Input: part model. Units: mm. Frame: model coordinates. A direction names the side the tool comes from. Give positions to 0.01 mm unless a question says otherwise; leave off trailing zeros. Write each loop counter-clockwise with the first axis right and the second up, starting at its lowest first coordinate (ties: lowest second). Pieces come first, ordered by that corner, then holes. Notation, with made-up numbers: (89, 14.5) - (121, 14.5) arc R22 cw to (121, 23.5) - close; hole circle Ø11 at (85.25, 72.5). An arc over 180 degrees is marked (long way). Answer as CSV lines item,"result".
```python
from build123d import *

# Parameters (mm, degrees)
BOSS_EXTRUDE4_DEPTH      = 4.2
BOSS_EXTRUDE4_DEPTH_BACK = 0.2
SKETCH10_R               = 5
BOSS_EXTRUDE5_DEPTH      = 9
SKETCH16_R               = 5
BOSS_EXTRUDE6_DEPTH      = 4.8
CUT_EXTRUDE2_DEPTH       = 20.805049861
HOLEWZD2_D               = 3.5
HOLEWZD2_DEPTH           = 1.8
CHAMFER2_SIZE            = 0.4


with BuildPart() as part:
    # Sketch10 → Boss-Extrude4 (new, two sides: drawn at the far end of the back side and taken through both)
    with BuildSketch(Plane.XY.offset(0.4).offset(-BOSS_EXTRUDE4_DEPTH_BACK)):
        with Locations((1, 0)):
            Circle(SKETCH10_R)
    extrude(amount=BOSS_EXTRUDE4_DEPTH + BOSS_EXTRUDE4_DEPTH_BACK)

    # Sketch11 → Boss-Extrude5 (add)
    with BuildSketch(Plane(origin=(0, 0, 0.2), x_dir=(-1, 0, 0), z_dir=(0, 0, -1))):
        with BuildLine():
            Line((-4, -3.05), (-4, 3.05))
            ThreePointArc((-4, 3.05), (-3.824264069, 3.474264069), (-3.4, 3.65))
            Line((-3.4, 3.65), (0, 3.65))
            ThreePointArc((0, 3.65), (3.65, 0), (0, -3.65))
            Line((0, -3.65), (-3.4, -3.65))
            ThreePointArc((-3.4, -3.65), (-3.824264069, -3.474264069), (-4, -3.05))
        make_face()
    extrude(amount=BOSS_EXTRUDE5_DEPTH)

    # Sketch16 → Boss-Extrude6 (add)
    with BuildSketch(Plane(origin=(0, 0, 4.6), x_dir=(-1, 0, 0), z_dir=(0, 0, -1))):
        with Locations((1, 0)):
            Circle(SKETCH16_R)
    extrude(amount=-BOSS_EXTRUDE6_DEPTH)

    # Sketch17 → Cut-Extrude2 (cut, through all)
    with BuildSketch(Plane.XY.offset(9.4)):
        with BuildLine():
            Line((2.2, -1.47732867), (2.2, 1.47732867))
            ThreePointArc((2.2, 1.47732867), (-2.65, 0), (2.2, -1.47732867))
        make_face()
    extrude(amount=-CUT_EXTRUDE2_DEPTH, mode=Mode.SUBTRACT)

    # HoleWzd2
    with Locations(Plane(origin=(4, 0, 0), x_dir=(0, 0, -1), z_dir=(1, 0, 0))):
        with Locations((5, 0)):
            Hole(HOLEWZD2_D / 2, depth=HOLEWZD2_DEPTH)

    # Chamfer2
    # the kernel refuses this chamfer: 0.4 mm, written as the material it takes off along each edge
    with BuildSketch(Plane(origin=(-1, 0, 9.4), x_dir=(-1, 0, 0), z_dir=(0, -1, 0))) as chamfer2_piece_1:
        Polygon((5, CHAMFER2_SIZE), (5 - CHAMFER2_SIZE, 0), (5, 0), align=None)
    revolve(axis=Axis((-1, 0, 9.4), (0, 0, -1)), mode=Mode.SUBTRACT)
    with BuildSketch(Plane(origin=(1, 0, 0.2), x_dir=(1, 0, 0), z_dir=(0, -1, 0))) as chamfer2_piece_2_section:
        Polygon((5, CHAMFER2_SIZE), (5 - CHAMFER2_SIZE, 0), (5, 0), align=None)
    chamfer2_piece_2 = revolve(axis=Axis((1, 0, 0.2), (0, 0, 1)), mode=Mode.PRIVATE)
    chamfer2_piece_2 = chamfer2_piece_2 - Plane(origin=(0, 0, 0.390166904), x_dir=(0, 1, 0), z_dir=(0, 0, 1)) * Cylinder(3.65, 20, mode=Mode.PRIVATE)
    add(chamfer2_piece_2, mode=Mode.SUBTRACT)


solid = part.part
```
Item 1: Mould query, pull axis Y, two halves, no side actions, for faces 1 (the face through (5.77, 1.5, 2.57)), 2 (the face through (3, 0, -8.8)), 3 (the face through (2.2, 0, 3)). Classes: +Y half, -Y half, draft (parallel to the pull), parting line (faces both ways), or undercut.
The answers:
face 1,"parting line"
face 2,"draft"
face 3,"undercut"
Item 2: Contact query for flat-ended pins moving along their axis: pin 1 (5.5 mm diameter, centred on y = 0, z = -5, fed in from -X); pin 2 (2.5 mm diameter, centred on y = -0.5, z = 0, fed in from -X); pin 3 (6 mm diameter, centred on x = 1, z = -1.5, fed in from +Y); pin 4 (3 mm diameter, centred on y = -4, z = -3, fed in from -X). Output: stop coordinate, or through.
The answers:
pin 1,"x = -3.65"
pin 2,"x = -4"
pin 3,"y = 5"
pin 4,"x = -2.66"
Item 3: Cut plane C-C on z = -5. Return the cut outline in (x, y), plus the area to 3 significant figures.
The answers:
outline,"(0, -3.65) - (3.4, -3.65) arc R0.6 ccw to (4, -3.05) - (4, -1.75) - (2.2, -1.75) - (2.2, -1.48) arc R2.65 cw (long way) to (2.2, 1.48) - (2.2, 1.75) - (4, 1.75) - (4, 3.05) arc R0.6 ccw to (3.4, 3.65) - (0, 3.65) arc R3.65 ccw to start"
area,"22.5 mm²"
Item 4: Cut plane D-D on z = 5.75. Return the cut outline in (x, y), plus the area to 3 significant figures.
The answers:
outline,"circle Ø10 at (-1, 0); hole (2.2, -1.48) - (2.2, 1.48) arc R2.65 ccw (long way) to start"
area,"57.4 mm²"
Item 5: Cut plane A-A on y = 0. Return the cut outline in (x, z), plus the area to 3 significant figures.
The answers:
outline,"(-6, 4.6) - (-4, 4.6) - (-4, 0.6) - (-3.65, 0.25) - (-3.65, -8.8) - (-2.65, -8.8) - (-2.65, 9.4) - (-5.6, 9.4) - (-6, 9) - close; (2.2, -8.8) - (4, -8.8) - (4, -6.75) - (2.2, -6.75) - close; (2.2, -3.25) - (4, -3.25) - (4, 0.2) - (5.6, 0.2) - (6, 0.6) - (6, 4.6) - (4, 4.6) - (4, 9) - (3.6, 9.4) - (2.2, 9.4) - close"
area,"66.0 mm²"
Item 6: Reachability of faces 4 (the face through (4.3, 0, 4.6)), 5 (the face through (2, 3.65, -4)), 6 (the face through (-4.3, 0, 4.6)) from +Z, -Z, +X, -X, +Y, -Y: full face, straight path, thin tool, end or side. Return the list, or none.
The answers:
face 4,"+Z, +X"
face 5,"-Z, +X, -X, +Y"
face 6,"-Z, -X"
Item 7: Cut plane B-B on z = -1. Return the cut outline in (x, y).
The answers:
outline,"(0, -3.65) - (3.4, -3.65) arc R0.6 ccw to (4, -3.05) - (4, 3.05) arc R0.6 ccw to (3.4, 3.65) - (0, 3.65) arc R3.65 ccw to start; hole (2.2, -1.48) - (2.2, 1.48) arc R2.65 ccw (long way) to start"
Item 8: Ray query, line 1 (X direction, y = 0, z = -3); line 2 (Y direction, x = 2.95, z = -5); line 3 (Z direction, x = -2.75, y = 4). Return the intervals inside material, ascending. Write a range as from..to.
The answers:
line 1,"-3.65..-2.65, 2.2..4"
line 2,"-3.65..-1.75, 1.75..3.65"
line 3,"4.6..9.4"
